Geometry check sheet. Reference: the model listing, model coordinates, mm. A direction names the side the tool comes from. Coordinates: 2 decimals unless noted, no trailing zeros. Loops run counter-clockwise (first coordinate to the right, second up) from the corner with the lowest first, then second, coordinate; pieces in that order, holes last. Notation, with made-up numbers: (22.25, -37.75) -> (64.25, -37.75) arc R8 ccw to (64.25, -29.75) -> close; hole circle Ø3 at (57.25, 52.25). An arc over 180 degrees is marked (long way). Answer as a JSON object with one key per item and string values.
from build123d import *

# Parameters (mm, degrees)
F0_R            = 118.6771656213
F1_DEPTH        = 6.35
F2_R            = 13.8727461935
F3_DEPTH        = 6.35
F3_COPIES_COUNT = 10
F5_DEPTH        = 12.7
F5_COPIES_COUNT = 22


# Not quite as in the source:
# - a pattern or mirror of a feature is missing from the dataset's text; its kind, count and spacing are read off the source's solid


with BuildPart() as f1:
    # F0 (on Front) → F1 (new body, symmetric)
    with BuildSketch(Plane.XZ):
        Circle(F0_R)
    extrude(amount=F1_DEPTH, both=True)

    # F2 (on face) → F3 (join)
    with BuildSketch(Plane.XZ.offset(6.35)):
        with Locations((-71.153357625, -68.4610754251)):
            Circle(F2_R)
    f3 = extrude(amount=F3_DEPTH)

    # F3_copies: F3 ×10 about axis
    f3_copies_axis = Axis((0, 0, 0), (0, 1, 0))
    for i in range(1, F3_COPIES_COUNT):
        add(f3.rotate(f3_copies_axis, i * 360 / F3_COPIES_COUNT))

    # F4 (on face) → F5 (join, through all)
    with BuildSketch(Plane.XZ.offset(6.35)):
        with BuildLine():
            Line((-135.5267614126, 0), (-117.5784646417, -16.1113094564))
            ThreePointArc((-117.5784646417, -16.1113094564), (-118.6661963279, -1.6135330732), (-117.9730534673, 12.9084582934))
            Line((-117.9730534673, 12.9084582934), (-135.5267614126, 0))
        make_face()
    f5 = extrude(amount=-F5_DEPTH)

    # F5_copies: F5 ×22 about axis
    f5_copies_axis = Axis((0, 0, 0), (0, 1, 0))
    for i in range(1, F5_COPIES_COUNT):
        add(f5.rotate(f5_copies_axis, i * 360 / F5_COPIES_COUNT))


solid = f1.part
1. Section check A-A, the plane x = -42. Record the boundary of the cut face in (y, z).
Evaluation:
{"outline": "(-12.7, 75) -> (-6.35, 75) -> (-6.35, -117.05) -> (6.35, -117.05) -> (6.35, 115.31) -> (-6.35, 115.31) -> (-6.35, 102.65) -> (-12.7, 102.65) -> close"}
2. Tool access check on faces 4 (the face through (98.528, -9.481, -54.377)), 5 (the face through (119.31, -0.09, 43.31)), 6 (the face through (-123.785, -0.089, 28.068)), 7 (the face through (46.65, -0.089, -117.903)). Record the directions out of +Z, -Z, +X, -X, +Y, -Y that give a thin tool (end or side, any length) a straight path to the whole face; none if there is none.
Evaluation:
{"face 4": "-Y", "face 5": "+X, +Y, -Y", "face 6": "-X, +Y, -Y", "face 7": "-Z, +Y, -Y"}
3. Depth check by flat-ended pin: P1, Ø1, axis at y = -10.5, z = -7, coming from the +X side; P2, Ø10, axis at x = -80, z = -33.5, coming from the -Y side; P3, Ø10, axis at y = -9, z = 37.5, coming from the +X side. Enter the tip coordinate at first touch or a pass-through.
Evaluation:
{"P1": "stops at x = -85.33", "P2": "stops at y = -6.35", "P3": "stops at x = 130.04"}
4. Mould release check, pull along X, two halves, no side actions. Record for faces 1 (the face through (-98, -12.7, -13)), 2 (the face through (110.064, -0.089, 62.954)), 3 (the face through (-43.249, -9.481, 74.954)): released by +X, released by -X, zero draft, split by the parting line, or undercut.
Evaluation:
{"face 1": "zero draft", "face 2": "released by +X", "face 3": "undercut"}
5. Thickness scan on probe 1 along Y at (x, z) = (-24, 63.5); probe 2 along Z at (x, y) = (70, -9.25); probe 3 along X at (y, z) = (4.5, 119). Record the ranges inside material, lowest first. Write a range as from..to.
Evaluation:
{"probe 1": "y = -6.35..6.35", "probe 2": "z = 54.64..82.29", "probe 3": "x = -57.64..-48.62, -29.4..-4.4, 1.17..27.39, 46.48..57.19"}
